Check sheet for the modelled part. Datum: model origin and axes. Units: mm. A direction names the side the tool comes from. Round coordinates to 2 decimals unless told otherwise and drop trailing zeros. Write each loop counter-clockwise with the first axis right and the second up, starting at its lowest first coordinate (ties: lowest second). Pieces come first, ordered by that corner, then holes. Notation, with made-up numbers: M 1,-15 L 22,-15 A24 ccw 22,-2 Z; hole C 73,-2 d2. An arc over 180 degrees is marked long. Put each result on its own line as item: value.
```python
from build123d import *

# Parameters (mm, degrees)
SKETCH_1_R          = 15
EXTRUDE_1_DEPTH     = 3
SKETCH_2_R          = 1.5
CUT_EXTRUDE_1_DEPTH = 22.424285286
SKETCH_5_R          = 5
EXTRUDE_2_DEPTH     = 30
SKETCH_7_R          = 7.5
EXTRUDE_4_DEPTH     = 15
CUT_EXTRUDE_START   = -15
CUT_EXTRUDE_2_DEPTH = 15
SKETCH_9_R          = 8.5
EXTRUDE_5_DEPTH     = 7


with BuildPart() as part:
    # 草图1 → 凸台-拉伸1 (new body)
    with BuildSketch(Plane.XY):
        Circle(SKETCH_1_R)
    extrude(amount=EXTRUDE_1_DEPTH)

    # 草图2 → 切除-拉伸1 (cut, through all)
    with BuildSketch(Plane.XY.offset(3)):
        with Locations((0, 12)):
            Circle(SKETCH_2_R)
        with Locations((12, 0)):
            Circle(SKETCH_2_R)
        with Locations((0, -12)):
            Circle(SKETCH_2_R)
        with Locations((-12, 0)):
            Circle(SKETCH_2_R)
    extrude(amount=-CUT_EXTRUDE_1_DEPTH, mode=Mode.SUBTRACT)

    # 草图5 → 凸台-拉伸2 (add)
    with BuildSketch(Plane.XY.offset(3)):
        Circle(SKETCH_5_R)
    extrude(amount=EXTRUDE_2_DEPTH)

    # 草图7 → 凸台-拉伸4 (add)
    with BuildSketch(Plane.XY.offset(3)):
        Circle(SKETCH_7_R)
    extrude(amount=EXTRUDE_4_DEPTH)

    # 草图8 → 切除-拉伸2 (cut)
    with BuildSketch(Plane.XY.offset(33).offset(CUT_EXTRUDE_START)):
        with BuildLine():
            Line((-3, 4), (3, 4))
            ThreePointArc((3, 4), (0, 5), (-3, 4))
        make_face()
    extrude(amount=CUT_EXTRUDE_2_DEPTH, mode=Mode.SUBTRACT)

    # 草图9 → 凸台-拉伸5 (add)
    with BuildSketch(Plane.XY.offset(3)):
        Circle(SKETCH_9_R)
    extrude(amount=EXTRUDE_5_DEPTH)


solid = part.part
```
1. Release check for a two-part mould opening along Y. For faces 1 (the flat face through (6.5, -6.5, 3)), 2 (the cylindrical face through (10.5, 0.07, 1.52)), 3 (the cylindrical face through (0, -5, 25)) record: +Y half, -Y half, draft (parallel to the pull), parting line (faces both ways), or undercut.
Computed values:
face 1: draft
face 2: undercut
face 3: parting line
2. Scan lines: probe 1 along Y at (x, z) = (0, 1.9); probe 2 along Y at (x, z) = (-12, 2.35); probe 3 along Z at (x, y) = (-5.75, -6.5). Record each from-to range of solid material in increasing order.
Computed values:
probe 1: y = -15 to -13.5, -10.5 to 10.5, 13.5 to 15
probe 2: y = -9 to -1.5, 1.5 to 9
probe 3: z = 0 to 3
3. Cross-section at A-A (y = 0). Enter the section's corners in (x, z).
Computed values:
outline: M -15,0 L -13.5,0 L -13.5,3 L -15,3 Z; M -10.5,0 L 10.5,0 L 10.5,3 L 8.5,3 L 8.5,10 L 7.5,10 L 7.5,18 L 5,18 L 5,33 L -5,33 L -5,18 L -7.5,18 L -7.5,10 L -8.5,10 L -8.5,3 L -10.5,3 Z; M 13.5,0 L 15,0 L 15,3 L 13.5,3 Z
4. Access from +Z, -Z, +X, -X, +Y, -Y to the whole of each face (thin tool, end or side, straight path). Record for faces 4 (the flat face through (0, 4, 25)), 5 (the flat face through (2, -5, 18)), 6 (the flat face through (0, 0, 0)).
Computed values:
face 4: +Z, +X, -X, +Y
face 5: +Z
face 6: -Z, +X, -X, +Y, -Y
5. Cross-section at C-C (x = -0.5). Enter the section's corners in (y, z).
Computed values:
outline: M -14.99,0 L -13.41,0 L -13.41,3 L -14.99,3 Z; M -10.59,0 L 10.59,0 L 10.59,3 L 8.49,3 L 8.49,10 L 7.48,10 L 7.48,18 L 4,18 L 4,33 L -4.97,33 L -4.97,18 L -7.48,18 L -7.48,10 L -8.49,10 L -8.49,3 L -10.59,3 Z; M 13.41,0 L 14.99,0 L 14.99,3 L 13.41,3 Z
6. Depth check by flat-ended pin: pin 1 Ø1.8 at (x, y) = (12, 0) entering from -Z; pin 2 Ø3.5 at (x, y) = (0, 12) entering from +Z; pin 3 Ø2 at (x, y) = (7, -1) entering from +Z; pin 4 Ø5 at (x, z) = (0.5, 24.5) entering from +Y. Enter the tip coordinate at first touch or a pass-through.
Computed values:
pin 1: passes through
pin 2: stops at z = 3
pin 3: stops at z = 18
pin 4: stops at y = 4
7. Cross-section at B-B (x = 12). Enter the section's corners in (y, z), then the cut area to 3 significant figures.
Computed values:
outline: M -9,0 L -1.5,0 L -1.5,3 L -9,3 Z; M 1.5,0 L 9,0 L 9,3 L 1.5,3 Z
area: 45.0 mm2
